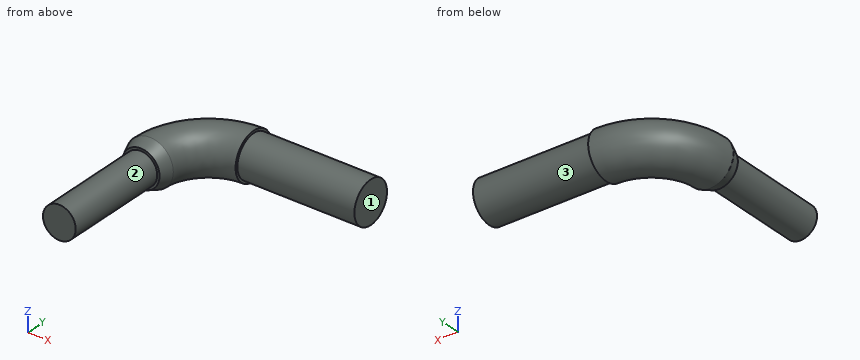
from build123d import *

# Parameters (mm, degrees)
F0_R     = 10
F3_ANGLE = 90
F4_R     = 7
F5_DEPTH = 50
F6_R     = 9
F7_DEPTH = 50
F8_DEPTH = 5
F9_SIZE2 = 4.99999
F9_SIZE  = 1.99999


# Not quite as in the source:
# - a fillet or chamfer is up to 0.001 mm smaller than in the source, because OpenCascade refuses the exact size


with BuildPart() as f3:
    # F0 (on Front) → F3 (revolve)
    with BuildSketch(Plane.XZ):
        with Locations((-40.3583608249, 0)):
            Circle(F0_R)
    revolve(axis=Axis((-15.3583608249, 0, 6.4160241745), (0, 0, -1)), revolution_arc=F3_ANGLE)

    # F6 (on face) → F7 (join)
    with BuildSketch(Plane.YZ.offset(-15.3583608249)):
        with Locations((25, 0)):
            Circle(F6_R)
    extrude(amount=F7_DEPTH)

    # F8 (add): a face of the model
    f8_faces = [f3.faces().sort_by_distance(p)[0] for p in [
        (-40.3583608249, 0, 0),
    ]]


with BuildPart() as f5:
    # F4 (on face) → F5 (new body)
    with BuildSketch(Plane.XZ):
        with Locations((-40.3583608249, 0)):
            Circle(F4_R)
    extrude(amount=F5_DEPTH)


with BuildPart() as f3_1:
    add(f3.part)

    add(f5.part)  # F8 merges F5
    extrude(f8_faces, amount=F8_DEPTH)

    # F9 (size 2 and 5 in the source; OpenCascade refuses exactly that, so slightly less here)
    f9_edges = [f3_1.edges().sort_by_distance(p)[0] for p in [
        (-50.358361, -5, 0),
    ]]
    f9_side = f3_1.faces().sort_by_distance((-50.075518, -5, 0))[0]
    chamfer(f9_edges, length=F9_SIZE, length2=F9_SIZE2, reference=f9_side)


solid = f3_1.part
Geometry: final body of the model. Coordinates: model frame, mm. Face numbers are marked on the shaded views. A direction names the side the tool comes from. Give positions to 0.01 mm unless a question says otherwise; leave off trailing zeros. Order: outer loops, then holes, each group sorted by start corner. A loop starts at its lowest first (then second) coordinate and runs counter-clockwise, first axis right, second up. Notation, with made-up numbers: (-7, -32.5) -> (23, -32.5) arc R16 ccw to (23, -26.5) -> close; hole circle Ø1 at (67.25, 41). An arc over 180 degrees is marked (long way). Put each result on its own line as item: value.
Q1. Section C-C, the plane y = -15.5. Return loops of the section in (x, z).
Here are the results:
outline: circle Ø14 at (-40.36, 0)
Q2. Material intervals for L1, parallel to Y at x = -36.5, z = -6.25; L2, parallel to Y at x = 22, z = 2; L3, parallel to X at y = 10, z = -4.25, sorted ascending.
Here are the results:
L1: y = -5 to 25.09
L2: y = 16.23 to 33.77
L3: x = -47.91 to -27.78
Q3. Section B-B, the plane x = 10.5. Return loops of the section in (y, z), then the cut area to 3 significant figures.
Here are the results:
outline: circle Ø18 at (25, 0)
area: 254 mm^2
Q4. Reachability of the marked faces 1, 2 and 3 from +Z, -Z, +X, -X, +Y, -Y: full face, straight path, thin tool, end or side. Return the list, or none.
Here are the results:
face 1: +Z, -Z, +X, +Y, -Y
face 2: -Y
face 3: +X
Q5. Pin query (flat end, axial travel): pin 1 (4 mm diameter, centred on y = -6, z = -2, fed in from -X); pin 2 (8 mm diameter, centred on x = -12.5, z = 6, fed in from -Y); pin 3 (4 mm diameter, centred on y = 9.5, z = -0.5, fed in from +X). Return the tip coordinate at first contact, or that it passes through.
Here are the results:
pin 1: stops at x = -48.61
pin 2: stops at y = 15.53
pin 3: stops at x = -25
